Input: dimensioned drawing with shaded views. Units: mm. Origin: part minimum x, y, z. A direction names the side the tool comes from. Round coordinates to 2 decimals unless told otherwise and drop trailing zeros. Order: outer loops, then holes, each group sorted by start corner. A loop starts at its lowest first (then second) coordinate and runs counter-clockwise, first axis right, second up. Notation, with made-up numbers: (22.25, 14) - (49.25, 14) arc R11 cw to (49.25, 21) - close; hole circle Ø10 at (-18, 21.5). An arc over 180 degrees is marked (long way). Return JSON: item names as keys, results as strings. Group by question number.
1) Access query for the marked faces 4 and 5. Directions: +Z, -Z, +X, -X, +Y, -Y. A direction counts if a zero-diameter tool reaches every point of the face in a straight line with its end or side. Return the directions, or none.
2) Ray query, line 1 (X direction, y = 21.5, z = 6); line 2 (Z direction, x = 26, y = 4.5); line 3 (X direction, y = 12.5, z = 10.75). Return the intervals inside material, ascending. Write a range as from..to.
3) Section A-A, the plane y = 20. Return loops of the section in (x, z) (1 decimal).
4) Section D-D, the plane y = 7.5. Return loops of the section in (x, z) (1 decimal).
5) Mould query, pull axis X, two halves, no side actions, for the marked faces 1, 2 and 3. Classes: pulls with the +X half, pulls with the -X half, needs draft (parallel to the pull), parting line crosses it, or undercut.
6) Contact query for flat-ended pins moving along their axis: P1, Ø4.5, axis at x = 23.5, y = 10, coming from the +Z side; P2, Ø4, axis at y = 4, z = 12, coming from the +X side; P3, Ø6, axis at x = 23.76, y = 21.81, coming from the -Z side. Output: stop coordinate, or through.
7) Section B-B, the plane z = 6.5. Return loops of the section in (x, y), plus the area to 3 significant figures.
8) Section C-C, the plane x = 25. Return loops of the section in (y, z), plus the area to 3 significant figures.
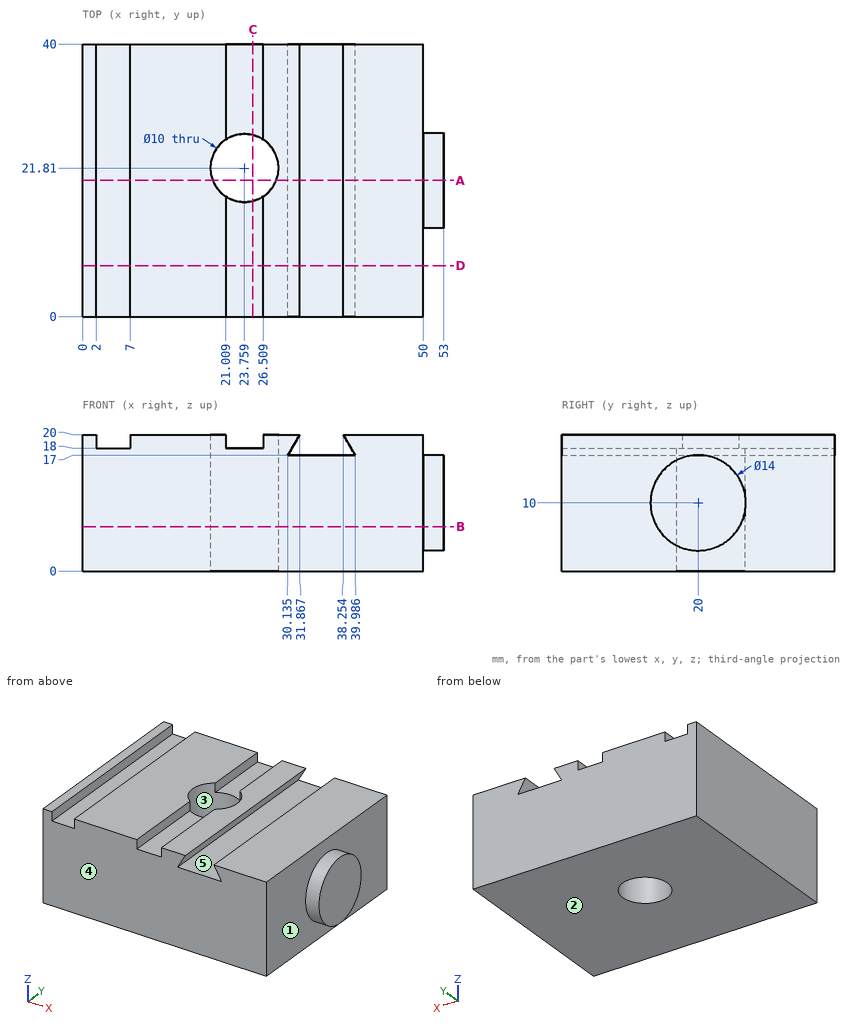
Geometry check:
{
 "1": {"face 4": "+Z, -Z, +X, -X, -Y", "face 5": "+Y, -Y"},
 "2": {"line 1": "0..18.77, 28.75..53", "line 2": "0..18", "line 3": "0..50"},
 "3": {"outline": "(0, 0) - (19.1, 0) - (19.1, 20) - (7, 20) - (7, 18) - (2, 18) - (2, 20) - (0, 20) - close; (28.4, 0) - (50, 0) - (50, 3) - (53, 3) - (53, 17) - (50, 17) - (50, 20) - (38.3, 20) - (40, 17) - (30.1, 17) - (31.9, 20) - (28.4, 20) - close"},
 "4": {"outline": "(0, 0) - (50, 0) - (50, 20) - (38.3, 20) - (40, 17) - (30.1, 17) - (31.9, 20) - (26.5, 20) - (26.5, 18) - (21, 18) - (21, 20) - (7, 20) - (7, 18) - (2, 18) - (2, 20) - (0, 20) - close"},
 "5": {"face 1": "pulls with the +X half", "face 2": "needs draft", "face 3": "undercut"},
 "6": {"P1": "z = 18", "P2": "x = 50", "P3": "through"},
 "7": {"outline": "(0, 0) - (50, 0) - (50, 13.94) - (53, 13.94) - (53, 26.06) - (50, 26.06) - (50, 40) - (0, 40) - close; hole circle Ø10 at (23.76, 21.81)", "area": "1,960 mm2"},
 "8": {"outline": "(0, 0) - (16.97, 0) - (16.97, 18) - (0, 18) - close; (26.65, 0) - (40, 0) - (40, 18) - (26.65, 18) - close", "area": "546 mm2"}
}
